Study the drawing (mm; zero at the part's minimum x, y, z) and answer. A direction names the side the tool comes from. Give positions to 0.01 mm unless a question says otherwise; leave off trailing zeros. Order: outer loops, then holes, each group sorted by start corner. A loop starts at its lowest first (then second) coordinate and runs counter-clockwise, first axis right, second up.
Item 1: Which of the six approach directions +Z, -Z, +X, -X, +Y, -Y give full straight-line access (tool end or side, diameter ignored) to the marked faces 1 and 2?
Item 2: A cutting plane is placed at B-B (y = 37.5). Write down the section's boundary in (x, z).
Item 3: A cutting plane is placed at C-C (x = 40). Write down the section's boundary in (y, z), plus the area to 3 significant figures.
Item 4: Find the intervals of material crossed by line 1 along Z through (x, y) = (40, 26.5); line 2 along X through (y, z) = (76, 93) (1 decimal); line 3 along X through (y, z) = (83.5, 135.5), in increasing order.
Item 5: Given pin 1 Ø4 at (x, z) = (31.5, 106) entering from -Y; pin 2 Ø1 at (x, z) = (46.5, 94) entering from +Y; pin 3 Ø5 at (y, z) = (69.5, 127) entering from +X, each flat-ended and moving along its own axis, determine where each tip first touches the part or whether it passes through.
Item 6: A cutting plane is placed at A-A (x = 72). Write down the section's boundary in (y, z).
Item 7: A cutting plane is placed at D-D (z = 268.5). Write down the section's boundary in (x, y).
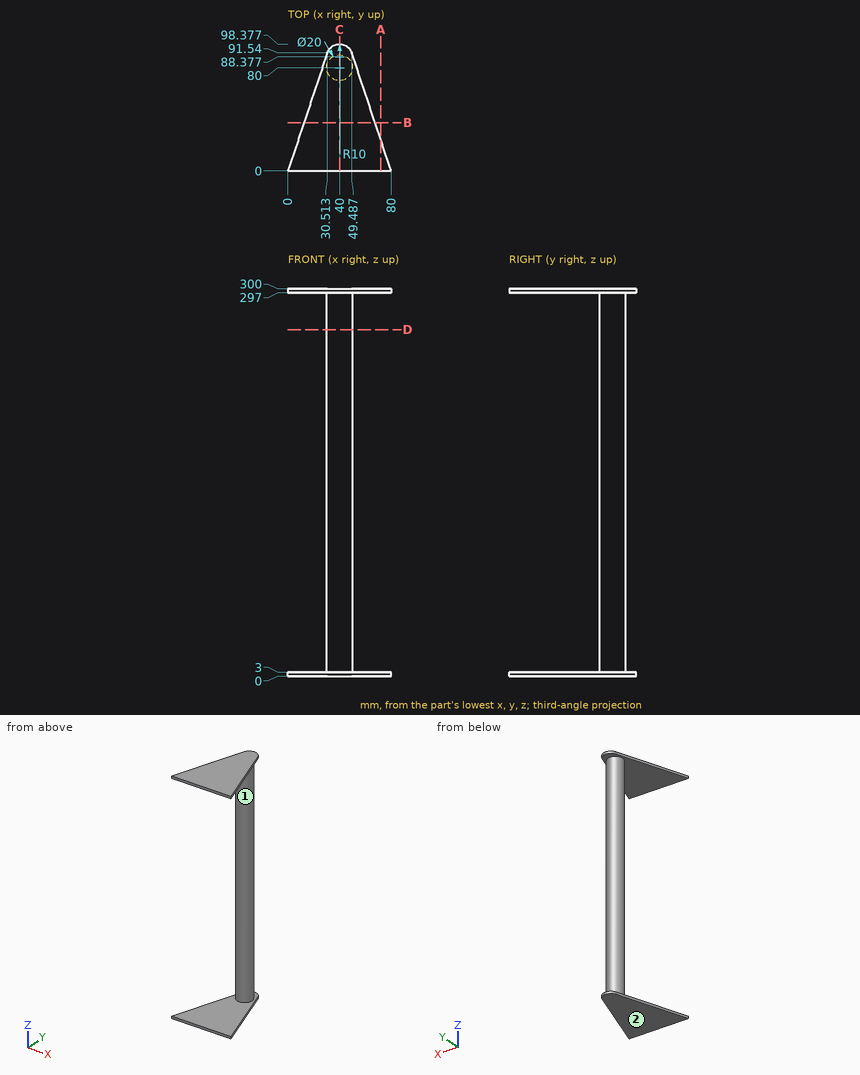
Response values:
1. face 1: none
1. face 2: -Z, +X, -X, +Y, -Y
2. outline: (12.5, 0) - (67.5, 0) - (67.5, 3) - (12.5, 3) - close; (12.5, 297) - (67.5, 297) - (67.5, 300) - (12.5, 300) - close
3. outline: (0, 0) - (98.38, 0) - (98.38, 3) - (90, 3) - (90, 297) - (98.38, 297) - (98.38, 300) - (0, 300) - (0, 297) - (70, 297) - (70, 3) - (0, 3) - close
3. area: 6,470 mm2
4. line 1: z = 0 to 3, 297 to 300
4. line 2: x = 30.8 to 49.2
4. line 3: x = 30.63 to 49.37
5. pin 1: stops at y = 72.4
5. pin 2: stops at y = 88
5. pin 3: stops at x = 46
6. outline: (0, 0) - (24, 0) - (24, 3) - (0, 3) - close; (0, 297) - (24, 297) - (24, 300) - (0, 300) - close
7. outline: circle Ø20 at (40, 80)
